The figure shows three views and two pictorial views of one solid part (mm, origin at its lowest corner). Answer the questions. A direction names the side the tool comes from. Give positions to 0.01 mm unless a question says otherwise; leave off trailing zeros. Write each loop counter-clockwise with the first axis right and the second up, starting at its lowest first coordinate (ties: lowest second). Pieces come first, ordered by that corner, then holes. Notation, with made-up numbers: M 43.5,-39.75 L 75.5,-39.75 A8 cw 75.5,-33.75 Z; hole C -23.5,76 d4. An arc over 180 degrees is marked long. Return JSON: item names as keys, results as strings.
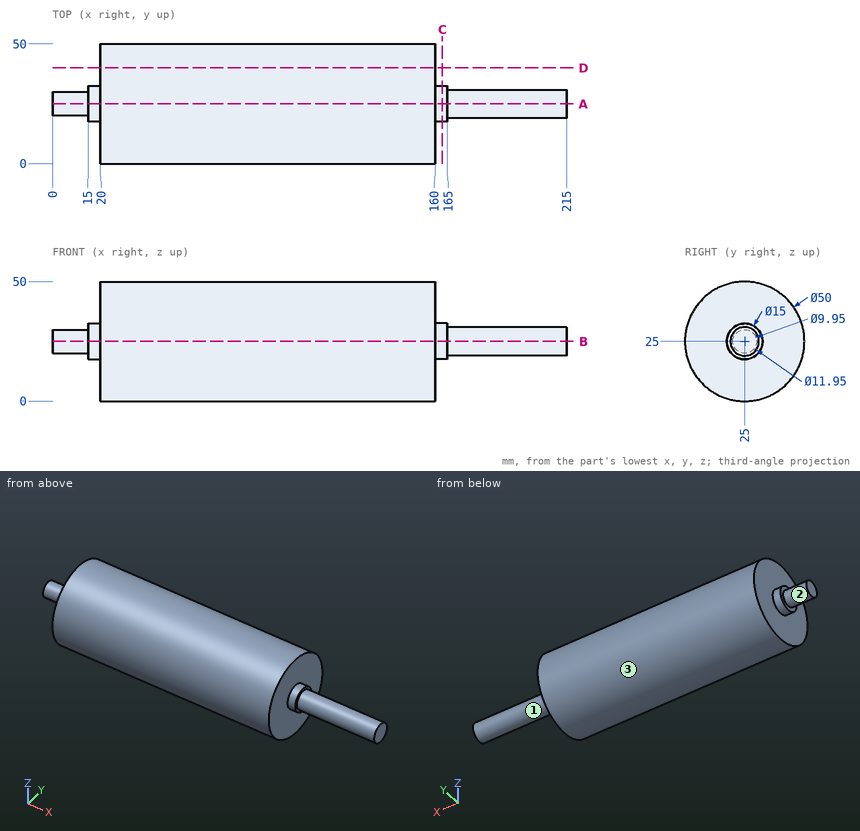
Item 1: A cutting plane is placed at C-C, the plane x = 163. Write down the section's boundary in (y, z).
Geometry results:
{"outline": "C 25,25 d15"}
Item 2: Given pin 1 Ø2 at (x, z) = (34, 21) entering from -Y; pin 2 Ø2 at (x, z) = (47.5, 11.5) entering from -Y; pin 3 Ø2 at (y, z) = (34.5, 39.5) entering from -X, each flat-ended and moving along its own axis, determine where each tip first touches the part or whether it passes through.
Geometry results:
{"pin 1": "stops at y = 0.18", "pin 2": "stops at y = 3.35", "pin 3": "stops at x = 20"}
Item 3: A cutting plane is placed at D-D, the plane y = 40. Write down the section's boundary in (x, z).
Geometry results:
{"outline": "M 20,5 L 160,5 L 160,45 L 20,45 Z"}
Item 4: Find the intervals of material crossed by line 1 (X direction, y = 20, z = 19.5); line 2 (X direction, y = 5.5, z = 33); line 3 (Y direction, x = 59.5, z = 24), in increasing order.
Geometry results:
{"line 1": "x = 15 to 165", "line 2": "x = 20 to 160", "line 3": "y = 0.02 to 49.98"}
Item 5: A cutting plane is placed at A-A, the plane y = 25. Write down the section's boundary in (x, z) (3 decimals), plus the area to 3 significant figures.
Geometry results:
{"outline": "M 0,20.025 L 15,20.025 L 15,17.5 L 20,17.5 L 20,0 L 160,0 L 160,17.5 L 165,17.5 L 165,19.025 L 215,19.025 L 215,30.975 L 165,30.975 L 165,32.5 L 160,32.5 L 160,50 L 20,50 L 20,32.5 L 15,32.5 L 15,29.975 L 0,29.975 Z", "area": "7,900 mm2"}
Item 6: Which of the six approach directions +Z, -Z, +X, -X, +Y, -Y give full straight-line access (tool end or side, diameter ignored) to the marked faces 1, 2 and 3?
Geometry results:
{"face 1": "+X", "face 2": "-X", "face 3": "+X, -X"}
